Print and shaded views of the part. All mm, measured from the part's lowest x, y and z. A direction names the side the tool comes from. Round coordinates to 2 decimals unless told otherwise and drop trailing zeros. Loops run counter-clockwise (first coordinate to the right, second up) from the corner with the lowest first, then second, coordinate; pieces in that order, holes last. Notation, with made-up numbers: (57, 70) -> (80, 70) arc R22 ccw to (80, 97) -> close; hole circle Ø8 at (-37, 64). An arc over 180 degrees is marked (long way). Answer as CSV lines item,"result".
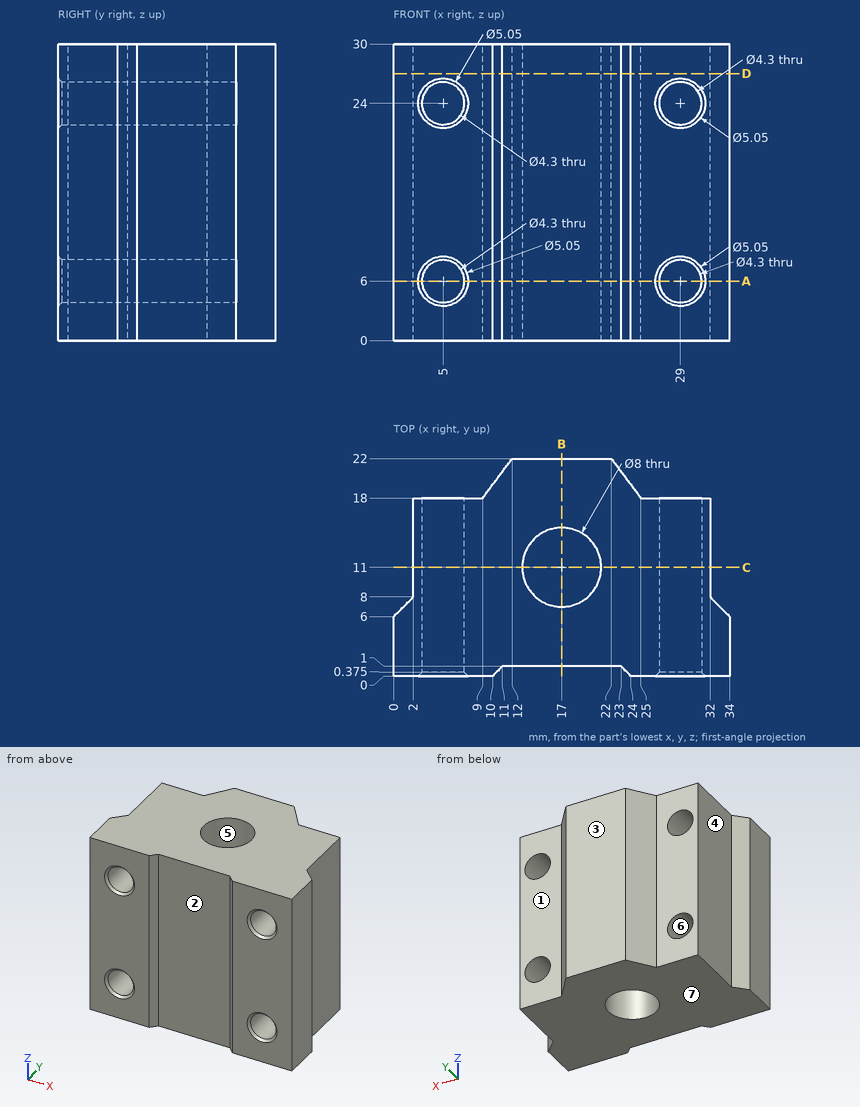
Q1. Drill centre lines: line 1 along Z through (x, y) = (5, 4.25); line 2 along Z through (x, y) = (30, 12); line 3 along X through (y, z) = (5.5, 6.5). Where is each one in solid material? Low to high.
Geometry results:
line 1,"0 to 3.85, 8.15 to 21.85, 26.15 to 30"
line 2,"0 to 4.1, 7.9 to 22.1, 25.9 to 30"
line 3,"0 to 2.91, 7.09 to 26.91, 31.09 to 34"
Q2. Saw through at A-A, the plane z = 6. Give the number of separate pieces and of enclosed holes in the cut face, then the cut area to 3 significant figures.
Geometry results:
separate pieces,"3"
enclosed holes,"1"
area,"402 mm2"
Q3. Saw through at C-C, the plane y = 11. Write the cut outline in (x, z), then the cut area to 3 significant figures.
Geometry results:
outline,"(2, 0) -> (13, 0) -> (13, 30) -> (2, 30) -> close; (21, 0) -> (32, 0) -> (32, 30) -> (21, 30) -> close; hole circle Ø4.3 at (5, 6); hole circle Ø4.3 at (5, 24); hole circle Ø4.3 at (29, 6); hole circle Ø4.3 at (29, 24)"
area,"602 mm2"
Q4. Drop flat-ended pins along their axis: P1, Ø2.5, axis at x = 29, z = 6, coming from the +Y side; P2, Ø1, axis at y = 18, z = 16.5, coming from the +X side; P3, Ø8, axis at x = 30.5, z = 25.5, coming from the +Y side; P4, Ø8, axis at y = 15, z = 14, coming from the -X side. Give the stop position or say it passes through.
Geometry results:
P1,"through"
P2,"x = 32"
P3,"y = 18"
P4,"x = 2"
Q5. Two-plate mould, pull along Z, no slides. Class the marked faces 5, 6 and 7: pulls with the +Z half, pulls with the -Z half, needs draft (parallel to the pull), parting line crosses it, or undercut.
Geometry results:
face 5,"needs draft"
face 6,"undercut"
face 7,"pulls with the -Z half"
Q6. Which spindle directions (+Z, -Z, +X, -X, +Y, -Y) get a long thin tool onto all of the face, cutting with end or side? Do the marked faces 1, 2, 3 and 4. Say none if no direction does.
Geometry results:
face 1,"+Z, -Z, +X, +Y"
face 2,"+Z, -Z, -Y"
face 3,"+Z, -Z, +X, -X, +Y"
face 4,"+Z, -Z, -X, +Y"
Q7. Saw through at B-B, the plane x = 17. Write the cut outline in (y, z), then the cut area to 3 significant figures.
Geometry results:
outline,"(1, 0) -> (7, 0) -> (7, 30) -> (1, 30) -> close; (15, 0) -> (22, 0) -> (22, 30) -> (15, 30) -> close"
area,"390 mm2"
Q8. Saw through at D-D, the plane z = 27. Write the cut outline in (x, y), then the cut area to 3 significant figures.
Geometry results:
outline,"(0, 0) -> (10, 0) -> (11, 1) -> (23, 1) -> (24, 0) -> (34, 0) -> (34, 6) -> (32, 8) -> (32, 18) -> (25, 18) -> (22, 22) -> (12, 22) -> (9, 18) -> (2, 18) -> (2, 8) -> (0, 6) -> close; hole circle Ø8 at (17, 11)"
area,"557 mm2"
